Build history of the part. All positions in model axes, mm. A direction names the side the tool comes from. Round coordinates to 2 decimals unless told otherwise and drop trailing zeros. Write each loop counter-clockwise with the first axis right and the second up, starting at its lowest first coordinate (ties: lowest second). Pieces come first, ordered by that corner, then holes.
Autodesk Inventor part; units mm, degrees
ref_plane "YZ Plane" through (0, 0, 0) normal (1, 0, 0) x (0, 1, 0)
ref_plane "XZ Plane" through (0, 0, 0) normal (0, 1, 0) x (-1, 0, 0)
ref_plane "XY Plane" through (0, 0, 0) normal (0, 0, 1) x (1, 0, 0)
ref_plane "Work Plane1" through (0, 0, 0) normal (0, 0, 1) x (1, 0, 0)
sketch "Sketch1" plane through (0, 0, 0) normal (0, 0, 1) x (1, 0, 0)
  circle A0 centre (-473.5705, 17.8) radius 2.5
  circle A1 centre (-473.5705, 17.8) radius 9.9 construction
  circle A2 centre (-473.5705, -25) radius 2.5
  circle A3 centre (-473.5705, -25) radius 9.9 construction
  line L0 (-473.5705, -25) -> (-473.5705, 17.8) construction
  circle A4 centre (-513.5705, 17.8) radius 2.5
  circle A5 centre (-513.5705, 17.8) radius 9.9 construction
  circle A6 centre (-513.5705, -25) radius 2.5
  circle A7 centre (-513.5705, -25) radius 9.9 construction
  line L1 (-513.5705, 17.8) -> (-513.5705, -25) construction
  line L2 (-513.5705, 17.8) -> (-473.5705, 17.8) construction
  line L3 (-513.5705, -25) -> (-473.5705, -25) construction
  line L4 (-463.6705, 18.91) -> (-463.6705, -34.9)
  line L5 (-463.6705, -34.9) -> (-523.4705, -34.9)
  line L6 (-523.4705, -34.9) -> (-523.4705, 18.91)
  line L7 (-519.0445, 27.8) -> (-468.0964, 27.8)
  line L8 (-463.6705, 27.8) -> (-453.6705, 27.8) construction
  line L9 (-452.9305, 18.91) -> (-463.6705, 18.91)
  line L10 (-534.2105, 28.86) -> (-534.2105, 18.91)
  line L11 (-534.2105, 18.91) -> (-523.4705, 18.91)
  circle A8 centre (-460.5505, 28.86) radius 2.75
  line L12 (-473.5705, -3.6) -> (-408.7211, -3.6) construction
  line L13 (-564.232, 28.86) -> (-376.8573, 28.86) construction
  arc A9 (-452.9305, 28.86) -> (-468.0964, 27.8) centre (-460.5505, 28.86) ccw
  line L14 (-493.5705, 27.8) -> (-493.5705, -34.9) construction
  line L15 (-452.9305, 28.86) -> (-452.9305, 18.91)
  circle A10 centre (-526.5905, 28.86) radius 2.75
  arc A11 (-519.0445, 27.8) -> (-534.2105, 28.86) centre (-526.5905, 28.86) ccw
  point P0 (0, 0)
  point P1 (-514.2552, 27.8)
  point P2 (-534.2105, 10.8915)
  dimension "d2" = 10
  dimension "d14" = 0
  dimension "d16" = 32.46
  dimension "d17" = 33.02
  dimension "d18" = 5.5
  dimension "d19" = 7.62
  dimension "d20" = 8.89
extrude "Extrusion1" add sketch "Sketch1" along normal blind 6.35
sketch "Sketch2" plane through (0, 0, 6.35) normal (0, 0, 1) x (1, 0, 0)
  line L0 (-463.6705, 18.91) -> (-452.9305, 18.91)
  line L1 (-452.9305, 18.91) -> (-463.6705, 8.17)
  line L2 (-534.2105, 28.86) -> (-534.2105, 18.91)
  line L3 (-534.2105, 18.91) -> (-523.4705, 8.17)
  line L4 (-523.4705, 18.91) -> (-523.4705, -34.9)
  line L5 (-534.2105, 18.91) -> (-523.4705, 18.91)
  line L6 (-534.2105, 18.91) -> (-523.4705, 18.91)
  line L7 (-523.4705, 8.17) -> (-523.4705, 18.91)
  line L8 (-463.6705, -34.9) -> (-463.6705, 18.91)
  line L9 (-463.6705, 8.17) -> (-463.6705, 18.91)
  line L10 (-452.9305, 18.91) -> (-463.6705, 18.91)
  point P0 (0, 0)
  point P1 (-548.4705, 27.8)
  point P2 (-548.4705, 15.264)
  dimension "d6" = 45
extrude "Extrusion2" add sketch "Sketch2" against normal up to surface (6.35 mm away)
properties part number "CarriagePlate"
1) Mould opens along X. For faces 4 (the cylindrical face through (-461.256, 36.447, 3.131)), 5 (the flat face through (-528.9, 13.6, 3.2)), 6 (the flat face through (-452.93, 24, 3)) say: released by +X, released by -X, zero draft, split by the parting line, or undercut.
Results:
face 4: undercut
face 5: released by -X
face 6: released by +X
2) Pin check, flat tips, straight feed: pin 1 Ø1.9 at (x, z) = (-504.5, 3.5) entering from +Y; pin 2 Ø2 at (y, z) = (12, 1) entering from -X; pin 3 Ø3 at (y, z) = (-7.5, 4) entering from -X. Stop position of each tip, or through.
Results:
pin 1: stops at y = 27.8
pin 2: stops at x = -528.3
pin 3: stops at x = -523.47
3) Slice it at D-D (x = -461.5). Write the cut outline in (y, z).
Results:
outline: (10.34, 0) - (26.28, 0) - (26.28, 6.35) - (10.34, 6.35) - close; (31.44, 0) - (36.42, 0) - (36.42, 6.35) - (31.44, 6.35) - close
4) Slice it at C-C (y = -25). Write the cut outline in (x, z).
Results:
outline: (-523.47, 0) - (-516.07, 0) - (-516.07, 6.35) - (-523.47, 6.35) - close; (-511.07, 0) - (-476.07, 0) - (-476.07, 6.35) - (-511.07, 6.35) - close; (-471.07, 0) - (-463.67, 0) - (-463.67, 6.35) - (-471.07, 6.35) - close
5) Wall check: L1, parallel to X at y = -23.5, z = 2; L2, parallel to Y at x = -458.5, z = 5.5; L3, parallel to Y at x = -507.5, z = 0.5. Give the ranges that are in metal, low to high.
Results:
L1: x = -523.47 to -515.57, -511.57 to -475.57, -471.57 to -463.67
L2: y = 13.34 to 27.03, 30.69 to 36.2
L3: y = -34.9 to 27.8
6) Slice it at B-B (x = -472.5). Write the cut outline in (y, z).
Results:
outline: (-34.9, 0) - (-27.26, 0) - (-27.26, 6.35) - (-34.9, 6.35) - close; (-22.74, 0) - (15.54, 0) - (15.54, 6.35) - (-22.74, 6.35) - close; (20.06, 0) - (27.8, 0) - (27.8, 6.35) - (20.06, 6.35) - close
7) Which spindle directions (+Z, -Z, +X, -X, +Y, -Y) get a long thin tool onto all of the face, cutting with end or side? Do faces 1 (the flat face through (-523.47, -14, 3)), 2 (the flat face through (-463.67, -13, 3)), 3 (the flat face through (-494, 1, 0)). Say none if no direction does.
Results:
face 1: +Z, -Z, -X, -Y
face 2: +Z, -Z, +X, -Y
face 3: -Z, +X, -X, +Y, -Y
8) Slice it at A-A (z = 2.5). Write the cut outline in (x, y), plus the area to 3 significant figures.
Results:
outline: (-534.21, 18.91) - (-523.47, 8.17) - (-523.47, -34.9) - (-463.67, -34.9) - (-463.67, 8.17) - (-452.93, 18.91) - (-452.93, 28.86) arc R7.62 ccw (long way) to (-468.1, 27.8) - (-519.04, 27.8) arc R7.62 ccw (long way) to (-534.21, 28.86) - close; hole circle Ø5.5 at (-526.59, 28.86); hole circle Ø5 at (-513.57, -25); hole circle Ø5 at (-513.57, 17.8); hole circle Ø5 at (-473.57, -25); hole circle Ø5 at (-473.57, 17.8); hole circle Ø5.5 at (-460.55, 28.86)
area: 4,140 mm2
